Here's the drawing with two shaded views (mm, measured from the low corner). I have some questions. A direction names the side the tool comes from. Coordinates: 2 decimals unless noted, no trailing zeros. Order: outer loops, then holes, each group sorted by start corner. A loop starts at its lowest first (then second) coordinate and runs counter-clockwise, first axis right, second up. Notation, with made-up numbers: (2, -7) -> (54, -7) arc R20 ccw to (54, 28) -> close; hole circle Ø1 at (58.5, -6.5). An arc over 180 degrees is marked (long way). Write item = value, one per line.
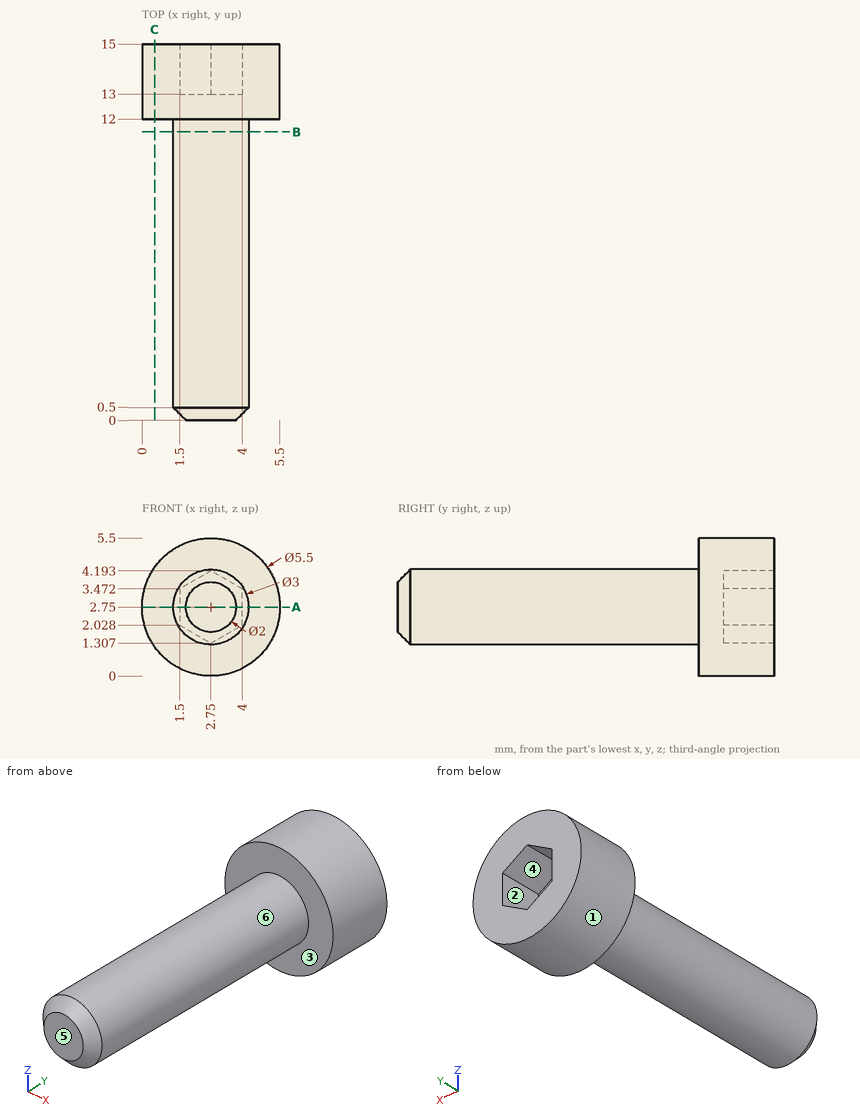
Item 1: I want a section at A-A, the plane z = 2.75. Please give me the cut outline in (x, y).
A:
outline = (0, 12) -> (1.25, 12) -> (1.25, 0.5) -> (1.75, 0) -> (3.75, 0) -> (4.25, 0.5) -> (4.25, 12) -> (5.5, 12) -> (5.5, 15) -> (4, 15) -> (4, 13) -> (1.5, 13) -> (1.5, 15) -> (0, 15) -> close
Item 2: For the marked faces 4, 5 and 6, which set-ups out of +Z, -Z, +X, -X, +Y, -Y let a thin tool reach every point of the face, with its end or its side?
A:
face_4 = +Y
face_5 = +Z, -Z, +X, -X, -Y
face_6 = -Y
Item 3: If I drill on probe 1 along Y at (x, z) = (2.7, 5); probe 2 along Y at (x, z) = (2.9, 1.8); probe 3 along X at (y, z) = (5, 1.6) (1 decimal), over which ranges is the centre line in solid material (lowest first)?
A:
probe_1 = 12 to 15
probe_2 = 0 to 13
probe_3 = 1.8 to 3.7
Item 4: I want a section at C-C, the plane x = 0.5. Please give me the cut outline in (y, z).
A:
outline = (12, 1.17) -> (15, 1.17) -> (15, 4.33) -> (12, 4.33) -> close
Item 5: I want a section at B-B, the plane y = 11.5. Please give me the cut outline in (x, z).
A:
outline = circle Ø3 at (2.75, 2.75)
Item 6: If we mould it in two halves opening along X, with no side actions, what happens to the marked faces 1, 2 and 3? For each: pulls with the +X half, pulls with the -X half, needs draft (parallel to the pull), parting line crosses it, or undercut.
A:
face_1 = parting line crosses it
face_2 = undercut
face_3 = needs draft
Item 7: I'm going to push flat-ended pins straight in: P1, Ø3, axis at x = 3.5, y = 2.5, coming from the -Z side; P2, Ø1, axis at x = 1, y = 6.5, coming from the +Z side; P3, Ø1.3, axis at x = 3, z = 2.5, coming from the +Y side. Where does each tip first touch, or does it pass through?
A:
P1 = 1.25
P2 = 3.58
P3 = 13
